Work out the finished part from the listing and answer in its coordinate system (mm). A direction names the side the tool comes from. Give positions to 0.01 mm unless a question says otherwise; leave off trailing zeros. Order: outer loops, then holes, each group sorted by start corner. A loop starts at its lowest first (then second) coordinate and runs counter-clockwise, first axis right, second up. Notation, with made-up numbers: (56.25, 17.5) - (82.25, 17.5) arc R13 ccw to (82.25, 22.5) - close; hole circle Ø11 at (-27.5, 18.25). An arc over 180 degrees is marked (long way). Put each result on its own line as item: value.
```python
from build123d import *

# Parameters (mm, degrees)
SKETCH1_W           = 114.3
SKETCH1_H           = 177.8
SKETCH1_W_2         = 101.6
SKETCH1_H_2         = 165.1
BOSS_EXTRUDE1_DEPTH = 4.7625
SKETCH2_W           = 12.38677804
SKETCH2_H           = 4.7625
SKETCH2_W_2         = 12.7
BOSS_EXTRUDE2_DEPTH = 4.7625
SKETCH3_W           = 12.7
SKETCH3_H           = 4.7625
BOSS_EXTRUDE3_DEPTH = 4.7625
FILLET1_R           = 2.54
SKETCH5_W           = 114.3
SKETCH5_H           = 12.7
SKETCH5_W_2         = 101.6
SKETCH5_H_2         = 5.08
BOSS_EXTRUDE5_DEPTH = 4.7625
FILLET3_R           = 2.54


with BuildPart() as part:
    # Sketch1 → Boss-Extrude1 (new body)
    with BuildSketch(Plane(origin=(0, 0, 0), x_dir=(1, 0, 0), z_dir=(0, 1, 0))):
        Rectangle(SKETCH1_W, SKETCH1_H)
        Rectangle(SKETCH1_W_2, SKETCH1_H_2, mode=Mode.SUBTRACT)
    extrude(amount=BOSS_EXTRUDE1_DEPTH)

    # Sketch2 → Boss-Extrude2 (add)
    with BuildSketch(Plane.XY.offset(88.9)):
        with Locations((-38.1, 2.38125)):
            Rectangle(SKETCH2_W, SKETCH2_H)
        with Locations((12.7, 2.38125)):
            Rectangle(SKETCH2_W_2, SKETCH2_H)
    extrude(amount=BOSS_EXTRUDE2_DEPTH)

    # Sketch3 → Boss-Extrude3 (add)
    with BuildSketch(Plane(origin=(0, 0, -88.9), x_dir=(-1, 0, 0), z_dir=(0, 0, -1))):
        with Locations((-38.1, 2.38125)):
            Rectangle(SKETCH3_W, SKETCH3_H)
        with Locations((12.7, 2.38125)):
            Rectangle(SKETCH3_W, SKETCH3_H)
    extrude(amount=BOSS_EXTRUDE3_DEPTH)

    # Fillet1
    fillet1_edges = [part.edges().sort_by_distance(p)[0] for p in [
        (50.8, 2.38125, 82.55),
        (50.8, 2.38125, -82.55),
        (-50.8, 2.38125, -82.55),
        (-50.8, 2.38125, 82.55),
    ]]
    fillet(fillet1_edges, radius=FILLET1_R)

    # Sketch5 → Boss-Extrude5 (add)
    with BuildSketch(Plane.XZ):
        Rectangle(SKETCH5_W, SKETCH5_H)
        Rectangle(SKETCH5_W_2, SKETCH5_H_2, mode=Mode.SUBTRACT)
    extrude(amount=-BOSS_EXTRUDE5_DEPTH)

    # Fillet3
    fillet3_edges = [part.edges().sort_by_distance(p)[0] for p in [
        (-50.8, 2.38125, 6.35),
        (-50.8, 2.38125, -6.35),
        (50.8, 2.38125, -6.35),
        (50.8, 2.38125, 6.35),
        (50.8, 2.38125, -2.54),
        (-50.8, 2.38125, -2.54),
        (-50.8, 2.38125, 2.54),
        (50.8, 2.38125, 2.54),
    ]]
    fillet(fillet3_edges, radius=FILLET3_R - 0.0001)  # a hair under: the kernel refuses the full size


solid = part.part
```
(1) Section D-D, the plane y = 1.7 is taken. Count the separate pieces of the cut face and the enclosed holes in it, then the cut area to 3 significant figures.
Geometry check:
separate pieces: 1
enclosed holes: 3
area: 4,580 mm²
(2) Given pin 1 (2.5 mm diameter, centred on x = 47, y = 2, fed in from +Z); pin 2 (2.5 mm diameter, centred on y = 1.5, z = -90.5, fed in from -X); pin 3 (2.5 mm diameter, centred on y = 1.5, z = -92.5, fed in from +X); pin 4 (1.5 mm diameter, centred on x = 1.5, z = 0, fed in from +Y), each flat-ended and moving along its own axis, determine where each tip first touches the part or whether it passes through.
Geometry check:
pin 1: stops at z = 88.9
pin 2: stops at x = -19.05
pin 3: stops at x = 44.45
pin 4: passes through
(3) Determine the mould class of faces 1 (the face through (12, 2, -88.9)), 2 (the face through (-44.293, 2, 91)), 3 (the face through (-51, 2, 88.9)), 4 (the face through (-50.8, 2, 45)) for opening direction Z: pulls with the +Z half, pulls with the -Z half, needs draft (parallel to the pull), parting line crosses it, or undercut.
Geometry check:
face 1: pulls with the -Z half
face 2: needs draft
face 3: pulls with the +Z half
face 4: undercut
(4) Section C-C, the plane x = -1.5 is taken. Write down the section's boundary in (y, z), then the cut area to 3 significant figures.
Geometry check:
outline: (0, -88.9) - (4.76, -88.9) - (4.76, -82.55) - (0, -82.55) - close; (0, -6.35) - (4.76, -6.35) - (4.76, -2.54) - (0, -2.54) - close; (0, 2.54) - (4.76, 2.54) - (4.76, 6.35) - (0, 6.35) - close; (0, 82.55) - (4.76, 82.55) - (4.76, 88.9) - (0, 88.9) - close
area: 96.8 mm²
(5) Section B-B, the plane x = 10 is taken. Write down the section's boundary in (y, z).
Geometry check:
outline: (0, -88.9) - (4.76, -88.9) - (4.76, -82.55) - (0, -82.55) - close; (0, -6.35) - (4.76, -6.35) - (4.76, -2.54) - (0, -2.54) - close; (0, 2.54) - (4.76, 2.54) - (4.76, 6.35) - (0, 6.35) - close; (0, 82.55) - (4.76, 82.55) - (4.76, 93.66) - (0, 93.66) - close
(6) A tool of negligible diameter and unlimited length cuts with its end or side. For faces 5 (the face through (-13, 2, 88.9)), 6 (the face through (-50.8, 2, -44)), 7 (the face through (-6.35, 2, -91)), from which of +Z, -Z, +X, -X, +Y, -Y can it reach the whole face along a straight path? Write none if from no direction.
Geometry check:
face 5: +Z, +Y, -Y
face 6: +Y, -Y
face 7: -Z, +Y, -Y
(7) Section A-A, the plane z = -41 is taken. Write down the section's boundary in (x, y), then the cut area to 3 significant figures.
Geometry check:
outline: (-57.15, 0) - (-50.8, 0) - (-50.8, 4.76) - (-57.15, 4.76) - close; (50.8, 0) - (57.15, 0) - (57.15, 4.76) - (50.8, 4.76) - close
area: 60.5 mm²
(8) Straight lines are drawn through the part: line 1 (Z direction, x = -48.5, y = 2.6); line 2 (Z direction, x = -27.5, y = 2.9); line 3 (X direction, y = 1.45, z = -37.5). For each, find the intervals that lie inside material, in ascending order.
Geometry check:
line 1: z = -88.9 to -82.54, -6.36 to -2.53, 2.53 to 6.36, 82.54 to 88.9
line 2: z = -88.9 to -82.55, -6.35 to -2.54, 2.54 to 6.35, 82.55 to 88.9
line 3: x = -57.15 to -50.8, 50.8 to 57.15
